```python
from build123d import *

# Parameters (mm, degrees)
BOSS_EXTRUDE1_DEPTH = 5
SKETCH2_R           = 1.6
CUT_EXTRUDE1_DEPTH  = 138.102151697
CHAMFER1_SIZE       = 1.5


with BuildPart() as part:
    # Sketch1 → Boss-Extrude1 (new body)
    with BuildSketch(Plane(origin=(0, 0, 0), x_dir=(1, 0, 0), z_dir=(0, 1, 0))):
        Polygon((0, -114), (-15.2, -114), (-15.2, -109), (-73, -109), (-73, -85.5), (-76, -85.5), (-76, -57), (-73, -57), (-73, -28.5), (-76, -28.5), (-76, 0), (-73, 0), (-73, 28.5), (-76, 28.5), (-76, 57), (-73, 57), (-73, 85.5), (-76, 85.5), (-76, 109), (-45.6, 109), (-45.6, 114), (-15.2, 114), (-15.2, 109), (0, 109), align=None)
    boss_extrude1 = extrude(amount=BOSS_EXTRUDE1_DEPTH)

    # Mirror1: Boss-Extrude1 across plane
    add(boss_extrude1.mirror(Plane(origin=(0, 5, 0), x_dir=(0, 0, 1), z_dir=(1, 0, 0))))

    # Sketch2 → Cut-Extrude1 (cut, through all)
    with BuildSketch(Plane(origin=(0, 5, 0), x_dir=(1, 0, 0), z_dir=(0, 1, 0))):
        with Locations(Location((0, 104, 0), (0, 0, 270))):
            Circle(SKETCH2_R)
        with Locations(Location((-35.5, 25.5, 0), (0, 0, 270))):
            Circle(SKETCH2_R)
        with Locations(Location((35.5, 25.5, 0), (0, 0, 270))):
            Circle(SKETCH2_R)
        with Locations(Location((-35.5, -103, 0), (0, 0, 270))):
            Circle(SKETCH2_R)
        with Locations(Location((35.5, -103, 0), (0, 0, 270))):
            Circle(SKETCH2_R)
    extrude(amount=-CUT_EXTRUDE1_DEPTH, mode=Mode.SUBTRACT)

    # Chamfer1
    chamfer1_edges = [part.edges().sort_by_distance(p)[0] for p in [
        (0, 5, -105.6),
        (35.5, 5, -27.1),
        (-35.5, 5, -27.1),
        (-35.5, 5, 101.4),
        (35.5, 5, 101.4),
    ]]
    chamfer(chamfer1_edges, length=CHAMFER1_SIZE)


solid = part.part
```
Read the model definition and answer for the solid it produces. Units are mm, in the model's axes. A direction names the side the tool comes from. Give positions to 0.01 mm unless a question says otherwise; leave off trailing zeros. Write each loop counter-clockwise with the first axis right and the second up, starting at its lowest first coordinate (ties: lowest second). Pieces come first, ordered by that corner, then holes. Notation, with made-up numbers: M 27,37.25 L 85,37.25 A23 ccw 85,62.25 Z; hole C 44.25,79 d8. An arc over 180 degrees is marked long. Put each result on its own line as item: value. Start each with the question number.
1. Which of the six approach directions +Z, -Z, +X, -X, +Y, -Y give full straight-line access (tool end or side, diameter ignored) to faces 1 (the flat face through (15.2, 2, 112)), 2 (the flat face through (45.6, 2, -111)), 3 (the flat face through (-44, 2, 109)), 4 (the flat face through (73, 2, -14))?
2. Each of these flat-tipped pins is pushed along its axis until it touches: pin 1 Ø3 at (x, z) = (35.5, 103) entering from +Y; pin 2 Ø2.5 at (y, z) = (2, 103) entering from -X; pin 3 Ø2.5 at (x, y) = (-75, 2) entering from +Z; pin 4 Ø0.9 at (x, y) = (-75, 2.5) entering from -Z. Where does it stop, or does it pass through?
3. For a pull along X with two mould halves and no side action, classify faces 5 (the flat face through (-15.2, 2, -112)), 6 (the flat face through (-73, 2, 97)), 7 (the flat face through (31, 2, -114)), 8 (the flat face through (0, 2, -109)) as released by +X, released by -X, zero draft, split by the parting line, or undercut.
4. Consider line 1 along X through (y, z) = (2.55, -25.5); line 2 along X through (y, z) = (1.35, -104); line 3 along Z through (x, y) = (8.5, 0.6). Determine where each line is inside the solid, lowest interval first.
5. The part is cut by section A-A, the plane y = 1.4. Give the number of separate pieces and of enclosed holes in the cut face, and give its area (3 significant figures).
6. The part is cut by section C-C, the plane z = 97. Give the vertices of the cut face in (x, y).
7. The part is cut by section B-B, the plane x = 55.5. Give the vertices of the cut face in (y, z), and give its area (3 significant figures).
Final values:
1. face 1: +Z, +X, +Y, -Y
1. face 2: -Z, +X, +Y, -Y
1. face 3: +Z, -X, +Y, -Y
1. face 4: +X, +Y, -Y
2. pin 1: passes through
2. pin 2: stops at x = -73
2. pin 3: stops at z = 85.5
2. pin 4: stops at z = -109
3. face 5: undercut
3. face 6: released by -X
3. face 7: zero draft
3. face 8: undercut
4. line 1: x = -73 to -37.1, -33.9 to 33.9, 37.1 to 73
4. line 2: x = -76 to -1.6, 1.6 to 76
4. line 3: z = -109 to 114
5. separate pieces: 1
5. enclosed holes: 5
5. area: 32,900 mm²
6. outline: M -73,0 L 73,0 L 73,5 L -73,5 Z
7. outline: M 0,-109 L 5,-109 L 5,109 L 0,109 Z
7. area: 1,090 mm²
